```python
from build123d import *

# Parameters (mm, degrees)
F0_W     = 20.5
F0_H     = 75
F1_DEPTH = 25
F2_R     = 8.5
F3_DEPTH = 10
F5_D     = 4.2
F6_R     = 6
F7_DEPTH = 25


with BuildPart() as f1:
    # F0 (on Top) → F1 (new body)
    with BuildSketch(Plane.XY):
        with Locations((-0.3433860838, 14.475764136)):
            Rectangle(F0_W, F0_H)
    extrude(amount=F1_DEPTH)

    # F2 (on face) → F3 (join)
    with BuildSketch(Plane.XY.offset(25)):
        with Locations((0, -11.024235864)):
            Circle(F2_R)
    extrude(amount=F3_DEPTH)

    # F5 (through all)
    with Locations(Plane.XY.offset(25)):
        with Locations((-4.5289483146, 40.0326289237), (5.268279344, 40.0625547821)):
            Hole(F5_D / 2)

    # F6 (on face) → F7 (cut)
    with BuildSketch(Plane.XY.offset(35)):
        with Locations((0, -11.024235864)):
            Circle(F6_R)
    extrude(amount=-F7_DEPTH, mode=Mode.SUBTRACT)


solid = f1.part
```
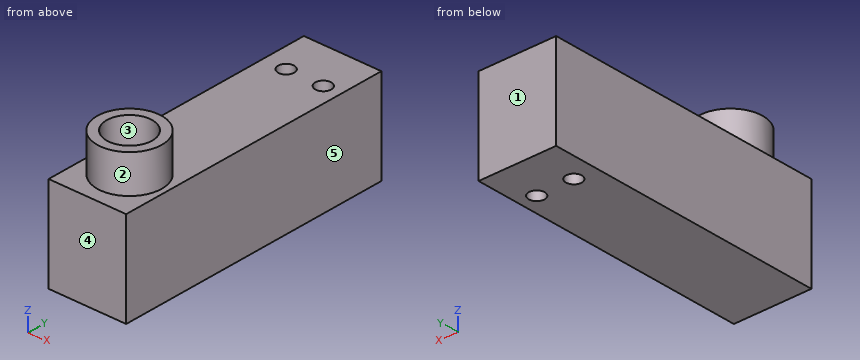
Design review of the part built by this model. Coordinates are the model's own, in mm. Face numbers are marked on the shaded views. A direction names the side the tool comes from. Round coordinates to 2 decimals unless told otherwise and drop trailing zeros. Order: outer loops, then holes, each group sorted by start corner. A loop starts at its lowest first (then second) coordinate and runs counter-clockwise, first axis right, second up. Notation, with made-up numbers: (-4, 54.5) - (6, 54.5) arc R32 cw to (6, 93.5) - close; hole circle Ø11 at (-15, 84). An arc over 180 degrees is marked (long way). Return JSON: item names as keys, results as strings.
Q1. The part is to be moulded in two halves that separate along X. For the marked faces 3, 4 and 5, say which applies: pulls with the +X half, pulls with the -X half, needs draft (parallel to the pull), parting line crosses it, or undercut.
Computed values:
{"face 3": "undercut", "face 4": "needs draft", "face 5": "pulls with the +X half"}
Q2. Machinability: for the marked faces 1 and 2, which of the approach directions +Z, -Z, +X, -X, +Y, -Y give a long, thin tool a straight path to every point of the face, cutting with its end or side? Answer none if there is none.
Computed values:
{"face 1": "+Z, -Z, +X, -X, +Y", "face 2": "+Z"}
Q3. Consider section C-C on z = 3. Write out the cut boundary in (x, y), plus the area to 3 significant figures.
Computed values:
{"outline": "(-10.59, -23.02) - (9.91, -23.02) - (9.91, 51.98) - (-10.59, 51.98) - close; hole circle Ø4.2 at (-4.53, 40.03); hole circle Ø4.2 at (5.27, 40.06)", "area": "1,510 mm2"}
Q4. Consider section A-A on x = -3.25. Write out the cut boundary in (y, z).
Computed values:
{"outline": "(-23.02, 0) - (38.37, 0) - (38.37, 25) - (-3.17, 25) - (-3.17, 35) - (-5.98, 35) - (-5.98, 10) - (-16.07, 10) - (-16.07, 35) - (-18.88, 35) - (-18.88, 25) - (-23.02, 25) - close; (41.7, 0) - (51.98, 0) - (51.98, 25) - (41.7, 25) - close"}
Q5. For pin 1 Ø11 at (x, y) = (0, -11.02) entering from +Z; pin 2 Ø5 at (y, z) = (13, 28) entering from -X; pin 3 Ø5.5 at (x, y) = (5.27, 40.06) entering from +Z, all flat-tipped, find the tip position at first contact; note any pin that passes through.
Computed values:
{"pin 1": "stops at z = 10", "pin 2": "passes through", "pin 3": "stops at z = 25"}
Q6. Consider section B-B on x = 0. Write out the cut boundary in (y, z), plus the area to 4 significant figures.
Computed values:
{"outline": "(-23.02, 0) - (51.98, 0) - (51.98, 25) - (-2.52, 25) - (-2.52, 35) - (-5.02, 35) - (-5.02, 10) - (-17.02, 10) - (-17.02, 35) - (-19.52, 35) - (-19.52, 25) - (-23.02, 25) - close", "area": "1,745 mm2"}
Q7. Consider section D-D on y = 15.5. Write out the cut boundary in (x, z), plus the area to 4 significant figures.
Computed values:
{"outline": "(-10.59, 0) - (9.91, 0) - (9.91, 25) - (-10.59, 25) - close", "area": "512.5 mm2"}
Q8. Wall thickness on L1, parallel to Y at x = 0, z = 19; L2, parallel to Y at x = 5.5, z = 7; L3, parallel to Z at x = -8.5, y = 38: over which ranges is each line inside the solid? List them lowest first. Write a range as [from, to].
Computed values:
{"L1": "y = [-23.02, -17.02], [-5.02, 51.98]", "L2": "y = [-23.02, 37.98], [42.15, 51.98]", "L3": "z = [0, 25]"}
